Answer from the drawing. Dimensions are ordinates in mm from the lowest x, y and z of the part. A direction names the side the tool comes from. Give positions to 0.01 mm unless a question says otherwise; leave off trailing zeros. Write each loop counter-clockwise with the first axis right and the second up, starting at its lowest first coordinate (ties: lowest second). Pieces come first, ordered by that corner, then holes.
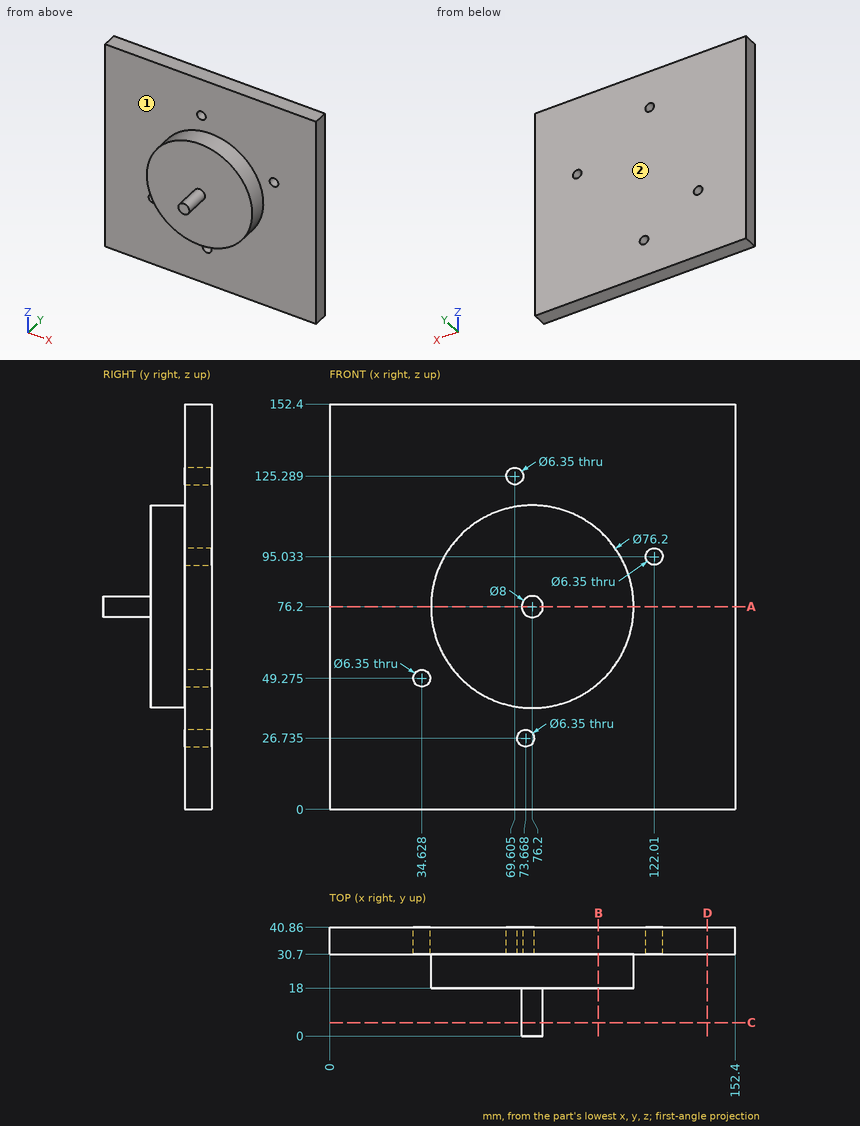
Item 1: A cutting plane is placed at C-C, the plane y = 5. Give the vertices of the cut face in (x, z), plus the area to 3 significant figures.
Conclusion:
outline: circle Ø8 at (76.2, 76.2)
area: 50.3 mm2
Item 2: Which of the six approach directions +Z, -Z, +X, -X, +Y, -Y give full straight-line access (tool end or side, diameter ignored) to the marked faces 1 and 2?
Conclusion:
face 1: -Y
face 2: +Z, -Z, +X, -X, +Y
Item 3: Consider probe 1 along Y at (x, z) = (39.5, 107.5); probe 2 along Z at (x, y) = (74.5, 22); probe 3 along X at (y, z) = (20.5, 74). Determine where each line is inside the solid, lowest interval first.
Conclusion:
probe 1: y = 30.7 to 40.86
probe 2: z = 38.14 to 114.26
probe 3: x = 38.16 to 114.24
Item 4: A cutting plane is placed at A-A, the plane z = 76.2. Give the vertices of the cut face in (x, y).
Conclusion:
outline: (0, 30.7) - (38.1, 30.7) - (38.1, 18) - (72.2, 18) - (72.2, 0) - (80.2, 0) - (80.2, 18) - (114.3, 18) - (114.3, 30.7) - (152.4, 30.7) - (152.4, 40.86) - (0, 40.86) - close
Item 5: A cutting plane is placed at B-B, the plane x = 101. Give the vertices of the cut face in (y, z).
Conclusion:
outline: (18, 47.28) - (30.7, 47.28) - (30.7, 0) - (40.86, 0) - (40.86, 152.4) - (30.7, 152.4) - (30.7, 105.12) - (18, 105.12) - close
Item 6: A cutting plane is placed at D-D, the plane x = 142. Give the vertices of the cut face in (y, z), plus the area to 3 significant figures.
Conclusion:
outline: (30.7, 0) - (40.86, 0) - (40.86, 152.4) - (30.7, 152.4) - close
area: 1,550 mm2
Item 7: Each of these flat-tipped pins is pushed along its axis until it touches: P1, Ø5, axis at x = 122.01, z = 95.03, coming from the +Y side; P2, Ø1.5, axis at x = 53.5, y = 28, coming from the -Z side; P3, Ø12, axis at y = 18, z = 95.5, coming from the -X side; P4, Ø7.5, axis at x = 73.67, z = 26.73, coming from the -Y side. Where does it stop, or does it pass through?
Conclusion:
P1: passes through
P2: stops at z = 45.06
P3: stops at x = 40.5
P4: stops at y = 30.7
